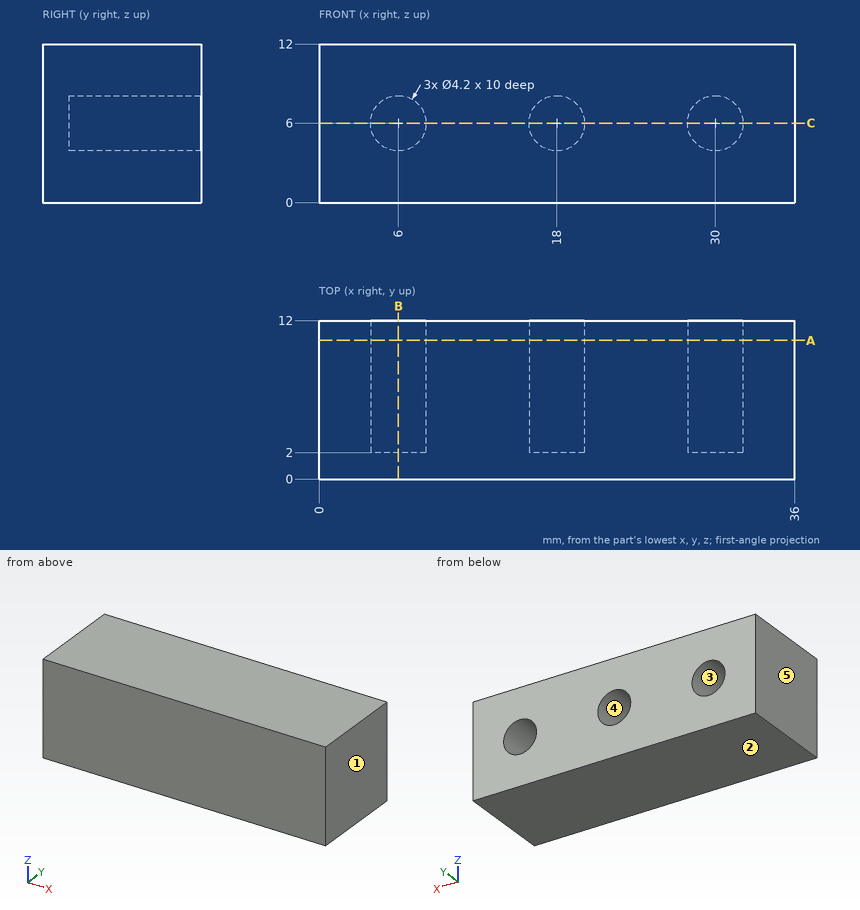
Check sheet for the drawn part. Datum: minimum x, y, z corner. Units: mm. A direction names the side the tool comes from. Give positions to 0.01 mm unless a question says otherwise; leave off trailing zeros. Order: outer loops, then holes, each group sorted by start corner. A loop starts at its lowest first (then second) coordinate and runs counter-clockwise, first axis right, second up.
1. Sectioned sample at C-C (z = 6). Record the boundary of the cut face in (x, y).
Completed:
outline: (0, 0) - (36, 0) - (36, 12) - (32.1, 12) - (32.1, 2) - (27.9, 2) - (27.9, 12) - (20.1, 12) - (20.1, 2) - (15.9, 2) - (15.9, 12) - (8.1, 12) - (8.1, 2) - (3.9, 2) - (3.9, 12) - (0, 12) - close
2. Draft check along X on the marked faces 1, 2 and 3. Enter one of: pulls with the +X half, pulls with the -X half, needs draft (parallel to the pull), parting line crosses it, or undercut.
Completed:
face 1: pulls with the +X half
face 2: needs draft
face 3: undercut
3. Sectioned sample at A-A (y = 10.5). Record the boundary of the cut face in (x, z), then the cut area to 3 significant figures.
Completed:
outline: (0, 0) - (36, 0) - (36, 12) - (0, 12) - close; hole circle Ø4.2 at (6, 6); hole circle Ø4.2 at (18, 6); hole circle Ø4.2 at (30, 6)
area: 390 mm2
4. Depth check by flat-ended pin: pin 1 (4 mm diameter, centred on x = 6, z = 6, fed in from -Y); pin 2 (2.5 mm diameter, centred on x = 30, z = 6, fed in from +Y). Enter the tip coordinate at first touch or a pass-through.
Completed:
pin 1: stops at y = 0
pin 2: stops at y = 2
5. Scan lines: line 1 (X direction, y = 6.25, z = 6); line 2 (X direction, y = 5.5, z = 5); line 3 (Y direction, x = 5.5, z = 6). Record each from-to range of solid material in increasing order.
Completed:
line 1: x = 0 to 3.9, 8.1 to 15.9, 20.1 to 27.9, 32.1 to 36
line 2: x = 0 to 4.15, 7.85 to 16.15, 19.85 to 28.15, 31.85 to 36
line 3: y = 0 to 2
6. Sectioned sample at B-B (x = 6). Record the boundary of the cut face in (y, z), then the cut area to 3 significant figures.
Completed:
outline: (0, 0) - (12, 0) - (12, 3.9) - (2, 3.9) - (2, 8.1) - (12, 8.1) - (12, 12) - (0, 12) - close
area: 102 mm2
7. Access from +Z, -Z, +X, -X, +Y, -Y to the whole of each face (thin tool, end or side, straight path). Record for the marked faces 4 and 5.
Completed:
face 4: +Y
face 5: +Z, -Z, -X, +Y, -Y
